Geometry check sheet. Reference: the model listing, model coordinates, mm. Face numbers are marked on the shaded views. A direction names the side the tool comes from. Coordinates: 2 decimals unless noted, no trailing zeros. Write each loop counter-clockwise with the first axis right and the second up, starting at its lowest first coordinate (ties: lowest second). Pieces come first, ordered by that corner, then holes. Notation, with made-up numbers: M 0,82 L 45,82 A30 ccw 45,116 Z; hole C 83,34.25 d7. An arc over 180 degrees is marked long. Put each result on its own line as item: value. Start each with the question number.
1) Cross-section at C-C on x = 73. Record the cut outline in (y, z).
2) Cross-section at A-A on y = 25.5. Record the cut outline in (x, z).
3) Set-up check for the marked faces 4, 5 and 6: record each of +Z, -Z, +X, -X, +Y, -Y from which the full face is reachable in a straight line by a thin tool's end or side.
4) Gauge pin test, flat ends, axial feed: pin 1 (15 mm diameter, centred on x = 85, z = 3, fed in from +Y); pin 2 (2.5 mm diameter, centred on x = 80, z = 24, fed in from +Y); pin 3 (2 mm diameter, centred on y = 26, z = 29.5, fed in from -X); pin 4 (1.5 mm diameter, centred on y = 6, z = 9, fed in from -X). Record the tip position at first contact, or that the pin passes through.
5) Cross-section at D-D on x = 82. Record the cut outline in (y, z).
6) Cross-section at B-B on z = 1. Record the cut outline in (x, y) (3 decimals), plus the area to 3 significant figures.
7) Scan lines: line 1 along Z through (x, y) = (81, 31); line 2 along Y through (x, z) = (87.5, 0); line 3 along Z through (x, y) = (82.5, 12.5). Record each from-to range of solid material in increasing order.
8) Mould release check, pull along Z, two halves, no side actions. Record for the marked faces 1, 2 and 3: released by +Z, released by -Z, zero draft, split by the parting line, or undercut.
from build123d import *

# Parameters (mm, degrees)
BOSS_EXTRUDE1_DEPTH = 11.5
BOSS_EXTRUDE2_DEPTH = 22
SKETCH3_R           = 2.5
CUT_EXTRUDE1_DEPTH  = 4
SKETCH4_R           = 4.5
CUT_EXTRUDE2_DEPTH  = 5
SKETCH5_R           = 2.75
CUT_EXTRUDE3_DEPTH  = 109.942645461
SKETCH6_R           = 2.75
CUT_EXTRUDE4_DEPTH  = 58.120859524
CUT_EXTRUDE5_DEPTH  = 8.2
SKETCH7_W           = 12
SKETCH7_H           = 11
CUT_EXTRUDE6_DEPTH  = 9.5
FILLET1_R           = 5.5
FILLET2_R           = 5


with BuildPart() as part:
    # Sketch1 → Boss-Extrude1 (new body)
    with BuildSketch(Plane(origin=(0, 0, 0), x_dir=(1, 0, 0), z_dir=(0, 1, 0))):
        with BuildLine():
            Line((67.071401597, -32.5), (94.571401597, -32.5))
            ThreePointArc((94.571401597, -32.5), (100, 0), (94.571401597, 32.5))
            Line((94.571401597, 32.5), (67.071401597, 32.5))
            ThreePointArc((67.071401597, 32.5), (74.530684367, 0), (67.071401597, -32.5))
        make_face()
    extrude(amount=BOSS_EXTRUDE1_DEPTH)

    # Sketch2 → Boss-Extrude2 (add)
    with BuildSketch(Plane.XZ.offset(-11.5)):
        with BuildLine():
            Line((81.240384046, 21), (87.515712875, 21))
            ThreePointArc((87.515712875, 21), (85.914014443, 26.810112315), (83.927051658, 32.5))
            Line((83.927051658, 32.5), (77.240384046, 32.5))
            Line((77.240384046, 32.5), (77.240384046, 25))
            ThreePointArc((77.240384046, 25), (78.411956922, 22.171572875), (81.240384046, 21))
        make_face()
        with BuildLine():
            Line((77.240384046, -25), (77.240384046, -32.5))
            Line((77.240384046, -32.5), (83.927051658, -32.5))
            ThreePointArc((83.927051658, -32.5), (85.914014443, -26.810112315), (87.515712875, -21))
            Line((87.515712875, -21), (81.240384046, -21))
            ThreePointArc((81.240384046, -21), (78.411956922, -22.171572875), (77.240384046, -25))
        make_face()
    extrude(amount=-BOSS_EXTRUDE2_DEPTH)

    # Sketch3 → Cut-Extrude1 (cut)
    with BuildSketch(Plane(origin=(0, 33.5, 0), x_dir=(1, 0, 0), z_dir=(0, 1, 0))):
        with Locations(Location((81.240384046, 25, 0), (0, 0, 270))):
            Circle(SKETCH3_R)
        with Locations(Location((81.240384046, -25, 0), (0, 0, 270))):
            Circle(SKETCH3_R)
    extrude(amount=-CUT_EXTRUDE1_DEPTH, mode=Mode.SUBTRACT)

    # Sketch4 → Cut-Extrude2 (cut)
    with BuildSketch(Plane.XZ):
        with Locations(Location((91.768319444, 24.5, 0), (0, 0, 270))):
            Circle(SKETCH4_R)
        with Locations(Location((91.768319444, -24.5, 0), (0, 0, 270))):
            Circle(SKETCH4_R)
    extrude(amount=-CUT_EXTRUDE2_DEPTH, mode=Mode.SUBTRACT)

    # Sketch5 → Cut-Extrude3 (cut, through all)
    with BuildSketch(Plane.XZ.offset(-5)):
        with Locations(Location((91.768319444, 24.5, 0), (0, 0, 270))):
            Circle(SKETCH5_R)
        with Locations(Location((91.768319444, -24.5, 0), (0, 0, 270))):
            Circle(SKETCH5_R)
    extrude(amount=-CUT_EXTRUDE3_DEPTH, mode=Mode.SUBTRACT)

    # Sketch6 → Cut-Extrude4 (cut, through all)
    with BuildSketch(Plane.ZY.offset(-67.071401597)):
        with Locations((0, 7.5)):
            Circle(SKETCH6_R)
    extrude(amount=-CUT_EXTRUDE4_DEPTH, mode=Mode.SUBTRACT)

    # Sketch8 → Cut-Extrude5 (cut)
    with BuildSketch(Plane(origin=(100, 0, 0), x_dir=(0, 0, -1), z_dir=(1, 0, 0))):
        with BuildLine():
            Line((-4.5, 7.5), (-4.5, 11.5))
            Line((-4.5, 11.5), (4.5, 11.5))
            Line((4.5, 11.5), (4.5, 7.5))
            ThreePointArc((4.5, 7.5), (0, 3), (-4.5, 7.5))
        make_face()
    extrude(amount=-CUT_EXTRUDE5_DEPTH, mode=Mode.SUBTRACT)

    # Sketch7 → Cut-Extrude6 (cut)
    with BuildSketch(Plane(origin=(0, 11.5, 0), x_dir=(1, 0, 0), z_dir=(0, 1, 0))):
        with Locations((77.8, 0)):
            Rectangle(SKETCH7_W, SKETCH7_H)
    extrude(amount=-CUT_EXTRUDE6_DEPTH, mode=Mode.SUBTRACT)

    # Fillet1
    # the kernel refuses this fillet: 5.5 mm, written as the material it adds along each edge
    with BuildSketch(Plane(origin=(60.577470777, 2, 5.5), x_dir=(0, 1, 0), z_dir=(1, 0, 0))) as fillet1_piece_1_section:
        with BuildLine():
            CenterArc((FILLET1_R, -FILLET1_R), FILLET1_R, 90, 90)
            Line((0, -FILLET1_R), (0, 0))
            Line((0, 0), (FILLET1_R, 0))
        make_face()
    fillet1_piece_1 = extrude(amount=36.972529223, mode=Mode.PRIVATE)
    fillet1_piece_1 = fillet1_piece_1 - Plane(origin=(0, 3.249781121, 0), x_dir=(0.899916620473715, 0, -0.43606200957566527), z_dir=(0, -1, 0)) * Cylinder(74.530684367, 96, mode=Mode.PRIVATE)
    add(fillet1_piece_1)
    with BuildSketch(Plane(origin=(97.55, 2, -5.5), x_dir=(0, 0, 1), z_dir=(-1, 0, 0))) as fillet1_piece_2_section:
        with BuildLine():
            CenterArc((FILLET1_R, FILLET1_R), FILLET1_R, 180, 90)
            Line((0, FILLET1_R), (0, 0))
            Line((0, 0), (FILLET1_R, 0))
        make_face()
    fillet1_piece_2 = extrude(amount=36.972529223, mode=Mode.PRIVATE)
    fillet1_piece_2 = fillet1_piece_2 - Plane(origin=(0, 3.245173128, 0), x_dir=(0.899916620473715, 0, -0.43606200957566527), z_dir=(0, -1, 0)) * Cylinder(74.530684367, 96, mode=Mode.PRIVATE)
    add(fillet1_piece_2)

    # Fillet2
    fillet2_edges = [part.edges().sort_by_distance(p)[0] for p in [
        (67.071401597, 5.75, 32.5),
        (67.071401597, 5.75, -32.5),
    ]]
    fillet(fillet2_edges, radius=FILLET2_R)


solid = part.part
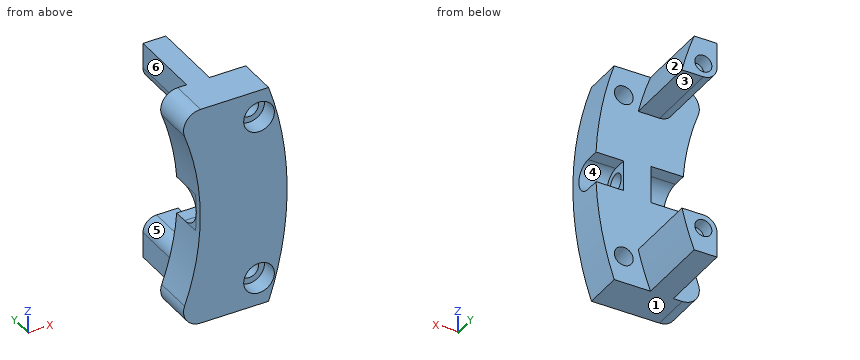
Answer key:
1. outline: M 0,-32.23 L 11.5,-32.23 L 11.5,-15.03 L 0,-15.03 Z; M 0,15.03 L 11.5,15.03 L 11.5,32.23 L 0,32.23 Z
2. outline: M 77.24,-32.5 L 83.93,-32.5 A90 ccw 87.52,-21 L 81.24,-21 A4 ccw 77.24,-25 Z; M 77.24,25 A4 ccw 81.24,21 L 87.52,21 A90 ccw 83.93,32.5 L 77.24,32.5 Z
3. face 4: +X, +Y
3. face 5: -X, +Y
3. face 6: +Z, -Z, -X, +Y
4. pin 1: stops at y = 11.5
4. pin 2: stops at y = 33.5
4. pin 3: stops at x = 77.24
4. pin 4: stops at x = 73.89
5. outline: M 0,-32.5 L 33.5,-32.5 L 33.5,-27.38 L 29.5,-27.38 L 29.5,-22.62 L 33.5,-22.62 L 33.5,-21 L 11.5,-21 L 11.5,-5.5 L 7.5,-5.5 A5.5 cw 7.5,5.5 L 11.5,5.5 L 11.5,21 L 33.5,21 L 33.5,22.62 L 29.5,22.62 L 29.5,27.38 L 33.5,27.38 L 33.5,32.5 L 0,32.5 Z
6. outline: M 74.524,0 L 99.995,0 L 99.995,3.113 L 91.8,3.113 L 91.8,4.938 L 83.8,4.938 L 83.8,2.092 L 74.524,2.092 Z; M 83.8,10.062 L 91.8,10.062 L 91.8,11.5 L 83.8,11.5 Z
6. area: 95.9 mm²
7. line 1: z = -32.5 to -27.49, -22.51 to -21.01, 21.01 to 22.51, 27.49 to 32.5
7. line 2: y = 0 to 4.75, 10.25 to 11.5
7. line 3: z = -32.5 to -21, 21 to 32.5
8. face 1: released by -Z
8. face 2: released by +Z
8. face 3: undercut
